Could you check a few things on this model? Use its own coordinates, in mm. Give positions to 0.01 mm unless a question says otherwise; leave off trailing zeros. Loops run counter-clockwise (first coordinate to the right, second up) from the corner with the lowest first, then second, coordinate; pieces in that order, holes last. Notation, with made-up numbers: M 62,38 L 90,38 A27 cw 90,71 Z; hole C 25,5.5 d7. An arc over 180 degrees is marked long. Use a Markdown table: item, result. Add a question column.
1) Suppose I cut it at B-B on x = 13.5. List the corners of the cut face in (y, z) for me, and give its area (3 significant figures).
2) We'd pull the mould along X, two halves only. Please class faces 1 (the flat face through (55.664, -38, 0)), 2 (the cylindrical face through (-30.283, -38.633, 17.221)), 3 (the flat face through (1, 0, 1)): +X half, -X half, draft (parallel to the pull), parting line (faces both ways), or undercut.
3) Suppose I cut it at A-A on z = 17.5. List the corners of the cut face in (x, y) for me.
4) If I drill on line 1 along Z through (x, y) = (13.5, -9); line 2 along X through (y, z) = (-49.5, -10); line 3 along Z through (x, y) = (-40, -15), over which ranges is the centre line in solid material (lowest first)? Write a range as [from, to].
5) Suppose I cut it at D-D on z = 12. List the corners of the cut face in (x, y) for me, and give its area (3 significant figures).
6) Will these pins go through, and if not, where does the flat tip stop? pin 1 Ø23.5 at (x, z) = (-11.93, 15) entering from +Y; pin 2 Ø13.5 at (x, z) = (13.47, 15) entering from -Y.
7) Suppose I cut it at C-C on y = -16.5. List the corners of the cut face in (x, z) for me.
```python
from build123d import *

# Parameters (mm, degrees)
F0_W     = 107.36537
F0_H     = 51.160677
F1_DEPTH = 76.2
F3_R     = 7.388078
F4_DEPTH = 84.074


with BuildPart() as f1:
    # F0 (on Front) → F1 (new body)
    with BuildSketch(Plane.XZ):
        with Locations((1.981586, 0.540432)):
            Rectangle(F0_W, F0_H)
    extrude(amount=F1_DEPTH)

    # F3 (on face) → F4 (cut)
    with BuildSketch(Plane.XZ.offset(76.2)):
        with Locations((-37.330247, 15.001875)):
            Circle(F3_R)
        with Locations((-37.330247, -10.398125)):
            Circle(F3_R)
        with Locations((-11.930247, 15.001875)):
            Circle(F3_R)
        with Locations((-11.930247, -10.398125)):
            Circle(F3_R)
        with Locations((13.469753, 15.001875)):
            Circle(F3_R)
        with Locations((13.469753, -10.398125)):
            Circle(F3_R)
    extrude(amount=-F4_DEPTH, mode=Mode.SUBTRACT)


solid = f1.part
```
Answer block:
| question | item | result |
|---|---|---|
| 1 | outline | M -76.2,-25.04 L 0,-25.04 L 0,-17.79 L -76.2,-17.79 Z; M -76.2,-3.01 L 0,-3.01 L 0,7.61 L -76.2,7.61 Z; M -76.2,22.39 L 0,22.39 L 0,26.12 L -76.2,26.12 Z |
| 1 | area | 1,650 mm^2 |
| 2 | face 1 | +X half |
| 2 | face 2 | undercut |
| 2 | face 3 | draft |
| 3 | outline | M -51.7,-76.2 L -44.28,-76.2 L -44.28,0 L -51.7,0 Z; M -30.38,-76.2 L -18.88,-76.2 L -18.88,0 L -30.38,0 Z; M -4.98,-76.2 L 6.52,-76.2 L 6.52,0 L -4.98,0 Z; M 20.42,-76.2 L 55.66,-76.2 L 55.66,0 L 20.42,0 Z |
| 4 | line 1 | z = [-25.04, -17.79], [-3.01, 7.61], [22.39, 26.12] |
| 4 | line 2 | x = [-51.7, -44.71], [-29.95, -19.31], [-4.55, 6.09], [20.85, 55.66] |
| 4 | line 3 | z = [-25.04, -17.29], [-3.51, 8.11], [21.89, 26.12] |
| 5 | outline | M -51.7,-76.2 L -44.08,-76.2 L -44.08,0 L -51.7,0 Z; M -30.58,-76.2 L -18.68,-76.2 L -18.68,0 L -30.58,0 Z; M -5.18,-76.2 L 6.72,-76.2 L 6.72,0 L -5.18,0 Z; M 20.22,-76.2 L 55.66,-76.2 L 55.66,0 L 20.22,0 Z |
| 5 | area | 5,090 mm^2 |
| 6 | pin 1 | stops at y = 0 |
| 6 | pin 2 | passes through |
| 7 | outline | M -51.7,-25.04 L 55.66,-25.04 L 55.66,26.12 L -51.7,26.12 Z; hole C -37.33,-10.4 d14.78; hole C -37.33,15 d14.78; hole C -11.93,-10.4 d14.78; hole C -11.93,15 d14.78; hole C 13.47,-10.4 d14.78; hole C 13.47,15 d14.78 |
